Job drawing, mm, ordinate dimensions from the low corner. One solid piece. Coordinates: 2 decimals unless noted, no trailing zeros. Order: outer loops, then holes, each group sorted by start corner. A loop starts at its lowest first (then second) coordinate and runs counter-clockwise, first axis right, second up. Notation, with made-up numbers: (-13, 37) - (35, 37) arc R16 cw to (35, 44) - close; hole circle Ø1 at (18, 4.5). An arc over 180 degrees is marked (long way). Return JSON: item names as keys, results as strings.
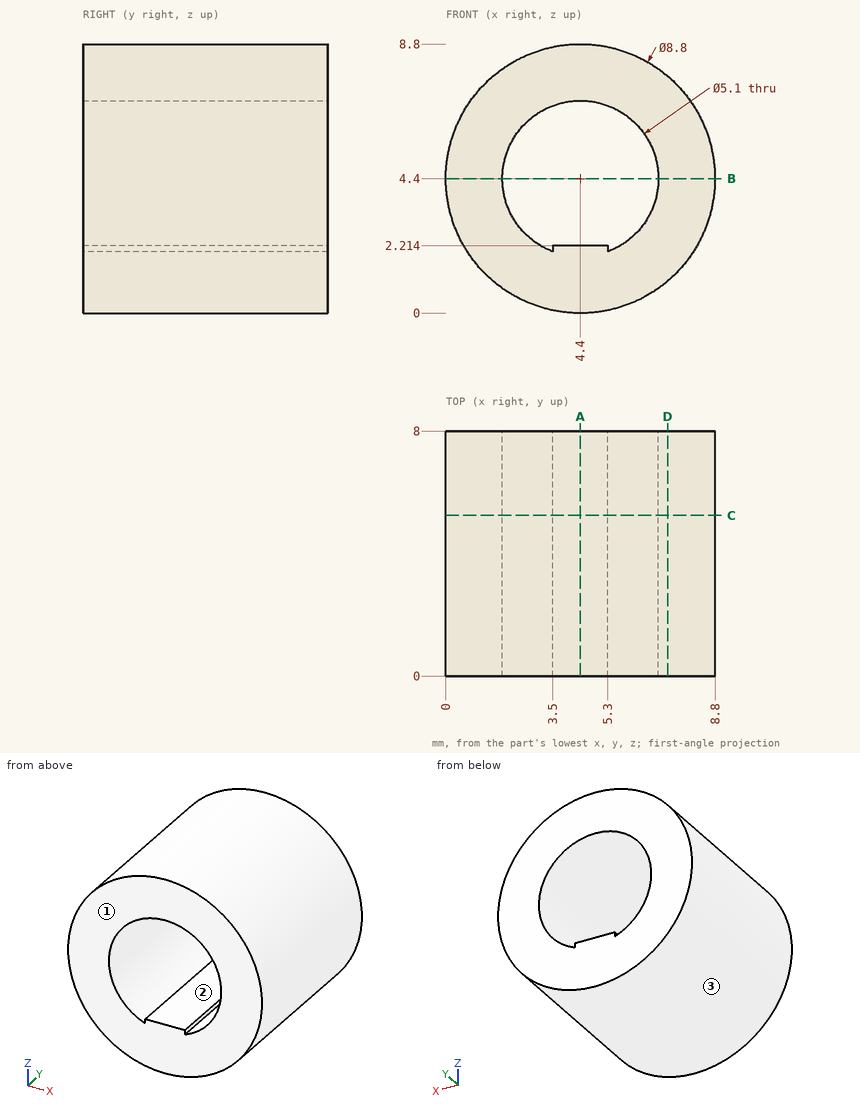
1. Mould opens along X. For the marked faces 1, 2 and 3 say: pulls with the +X half, pulls with the -X half, needs draft (parallel to the pull), parting line crosses it, or undercut.
Check values:
{"face 1": "needs draft", "face 2": "undercut", "face 3": "parting line crosses it"}
2. Drop flat-ended pins along their axis: pin 1 (1.5 mm diameter, centred on y = 5.5, z = 4, fed in from -X); pin 2 (2 mm diameter, centred on y = 5.5, z = 2, fed in from +X); pin 3 (4 mm diameter, centred on y = 5, z = 2, fed in from +X). Give the stop position or say it passes through.
Check values:
{"pin 1": "x = 0", "pin 2": "x = 8.57", "pin 3": "x = 8.78"}
3. Cut at A-A on x = 4.4. Give the cut face in (y, z).
Check values:
{"outline": "(0, 0) - (8, 0) - (8, 2.21) - (0, 2.21) - close; (0, 6.95) - (8, 6.95) - (8, 8.8) - (0, 8.8) - close"}
4. Cut at C-C on y = 5.25. Give the cut face in (x, z).
Check values:
{"outline": "circle Ø8.8 at (4.4, 4.4); hole (3.5, 2.01) - (3.5, 2.21) - (5.3, 2.21) - (5.3, 2.01) arc R2.55 ccw (long way) to start"}
5. Cut at B-B on z = 4.4. Give the cut face in (x, y), plus the area to 3 significant figures.
Check values:
{"outline": "(0, 0) - (1.85, 0) - (1.85, 8) - (0, 8) - close; (6.95, 0) - (8.8, 0) - (8.8, 8) - (6.95, 8) - close", "area": "29.6 mm²"}
6. Cut at D-D on x = 7.25. Give the cut face in (y, z), plus the area to 3 significant figures.
Check values:
{"outline": "(0, 1.05) - (8, 1.05) - (8, 7.75) - (0, 7.75) - close", "area": "53.6 mm²"}
7. Probe L1, parallel to X at y = 3.75, z = 4.4; L2, parallel to Z at x = 5.5, y = 3.75; L3, parallel to Z at x = 2.5, y = 2.75. List the from-to ranges inside material, lowest first.
Check values:
{"L1": "0 to 1.85, 6.95 to 8.8", "L2": "0.14 to 2.1, 6.7 to 8.66", "L3": "0.43 to 2.7, 6.1 to 8.37"}
